```python
from build123d import *

# Parameters (mm, degrees)
BOSS_EXTRUDE3_DEPTH     = 1
SKETCH2_W               = 8
SKETCH2_H               = 2
BOSS_EXTRUDE4_DEPTH     = 20
SKETCH5_R               = 1.5
CUT_EXTRUDE1_DEPTH      = 2
MIRROR2_COPY_1_SKETCH_W = 8
MIRROR2_COPY_1_SKETCH_H = 2
MIRROR2_COPY_1_DEPTH    = 20
MIRROR2_COPY_2_SKETCH_R = 1.5
MIRROR2_COPY_2_DEPTH    = 2


with BuildPart() as part:
    # Sketch1 → Boss-Extrude3 (new, symmetric)
    with BuildSketch(Plane.XY):
        with BuildLine():
            Line((-50, 17.5), (50, 17.5))
            ThreePointArc((50, 17.5), (67.5, 0), (50, -17.5))
            Line((50, -17.5), (-50, -17.5))
            ThreePointArc((-50, -17.5), (-67.5, 0), (-50, 17.5))
        make_face()
    extrude(amount=BOSS_EXTRUDE3_DEPTH, both=True)

    # Sketch2 → Boss-Extrude4 (add)
    with BuildSketch(Plane.XY.offset(1)):
        with Locations((-50, 9.6)):
            Rectangle(SKETCH2_W, SKETCH2_H)
    boss_extrude4 = extrude(amount=BOSS_EXTRUDE4_DEPTH)

    # Sketch5 → Cut-Extrude1 (cut)
    with BuildSketch(Plane.XZ.offset(-8.6)):
        with Locations(Location((-50, 13, 0), (0, 0, 270))):
            Circle(SKETCH5_R)
        with BuildLine():
            Line((-54, 13), (-54, 21))
            Line((-54, 21), (-46, 21))
            Line((-46, 21), (-46, 13))
            ThreePointArc((-46, 13), (-50, 17), (-54, 13))
        make_face()
    cut_extrude1 = extrude(amount=-CUT_EXTRUDE1_DEPTH, mode=Mode.SUBTRACT)

    # Mirror1: Boss-Extrude4, Cut-Extrude1 across plane
    add(boss_extrude4.mirror(Plane.ZX))
    add(cut_extrude1.mirror(Plane.ZX), mode=Mode.SUBTRACT)

    # Mirror2: Boss-Extrude4, Cut-Extrude1 across plane
    add(boss_extrude4.mirror(Plane(origin=(0, 0, 0), x_dir=(0, 0, 1), z_dir=(1, 0, 0))))
    add(cut_extrude1.mirror(Plane(origin=(0, 0, 0), x_dir=(0, 0, 1), z_dir=(1, 0, 0))), mode=Mode.SUBTRACT)

    # Mirror2 copy 1 sketch → Mirror2 copy 1 (add)
    with BuildSketch(Plane(origin=(0, 0, 1), x_dir=(-1, 0, 0), z_dir=(0, 0, 1))):
        with Locations((-50, 9.6)):
            Rectangle(MIRROR2_COPY_1_SKETCH_W, MIRROR2_COPY_1_SKETCH_H)
    extrude(amount=MIRROR2_COPY_1_DEPTH)

    # Mirror2 copy 2 sketch → Mirror2 copy 2 (cut)
    with BuildSketch(Plane(origin=(0, -8.6, 0), x_dir=(-1, 0, 0), z_dir=(0, 1, 0))):
        with Locations(Location((-50, 13, 0), (0, 0, 270))):
            Circle(MIRROR2_COPY_2_SKETCH_R)
        with BuildLine():
            Line((-54, 13), (-54, 21))
            Line((-54, 21), (-46, 21))
            Line((-46, 21), (-46, 13))
            ThreePointArc((-46, 13), (-50, 17), (-54, 13))
        make_face()
    extrude(amount=-MIRROR2_COPY_2_DEPTH, mode=Mode.SUBTRACT)


solid = part.part
```
Could you check a few things on this model? Use its own coordinates, in mm. A direction names the side the tool comes from. Coordinates: 2 decimals unless noted, no trailing zeros. Write each loop counter-clockwise with the first axis right and the second up, starting at its lowest first coordinate (ties: lowest second). Pieces come first, ordered by that corner, then holes. Notation, with made-up numbers: M -22.75,68 L 10.25,68 A5 cw 10.25,72 Z; hole C -8,81.25 d2. An arc over 180 degrees is marked long. Answer as CSV lines item,"result". Start each with the question number.
1) I want a section at C-C, the plane x = 27. Please give me the cut outline in (y, z).
2) We'd pull the mould along Y, two halves only. Please class faces 4 (the flat face through (-50, 10.6, 9)), 5 (the cylindrical face through (51.464, -9.586, 13.325)), 6 (the flat face through (-50, 8.6, 9)): +Y half, -Y half, draft (parallel to the pull), parting line (faces both ways), or undercut.
3) Please list where these lines run through material, in increasing order: line 1 (X direction, y = 9.1, z = 13); line 2 (Z direction, x = 50, y = 9); line 3 (Y direction, x = 50.5, z = 8). Write a range as from..to.
4) I want a section at B-B, the plane y = 14. Please give me the cut outline in (x, z).
5) For P1, Ø2, axis at y = 9.5, z = 8.5, coming from the -X side; P2, Ø6, axis at x = -47.5, z = 10, coming from the +Y side; P3, Ø17.5, axis at x = 3, y = -6.5, coming from the +Z side; P4, Ø1.8, axis at x = 50, z = 13, coming from the +Y side, each with a flat end and sliding along its axis, tell me the tip position at first contact or that it passes through.
6) For faces 1 (the flat face through (-50, -10.6, 9)), 2 (the flat face through (50, 10.6, 9)), 3 (the flat face through (50, 8.6, 9)), which set-ups out of +Z, -Z, +X, -X, +Y, -Y let a thin tool reach every point of the face, with its end or its side?
7) I want a section at A-A, the plane z = 4.75. Please give me the cut outline in (x, y), and give its area (3 significant figures).
Data:
1,outline,"M -17.5,-1 L 17.5,-1 L 17.5,1 L -17.5,1 Z"
2,face 4,"+Y half"
2,face 5,"draft"
2,face 6,"undercut"
3,line 1,"x = -54..-51.5, -48.5..-46, 46..48.5, 51.5..54"
3,line 2,"z = -1..11.5, 14.5..17"
3,line 3,"y = -10.6..-8.6, 8.6..10.6"
4,outline,"M -60.5,-1 L 60.5,-1 L 60.5,1 L -60.5,1 Z"
5,P1,"stops at x = -54"
5,P2,"stops at y = 10.6"
5,P3,"stops at z = 1"
5,P4,"passes through"
6,face 1,"+Z, +X, -X, -Y"
6,face 2,"+Z, +X, -X, +Y"
6,face 3,"+Z, +X, -X"
7,outline,"M -54,-10.6 L -46,-10.6 L -46,-8.6 L -54,-8.6 Z; M -54,8.6 L -46,8.6 L -46,10.6 L -54,10.6 Z; M 46,-10.6 L 54,-10.6 L 54,-8.6 L 46,-8.6 Z; M 46,8.6 L 54,8.6 L 54,10.6 L 46,10.6 Z"
7,area,"64.0 mm^2"
